Source: CAD feature listing. Evaluate the final solid. Frame: model axes, mm. Face numbers are marked on the shaded views. Coordinates: 2 decimals unless noted, no trailing zeros. Loops run counter-clockwise (first coordinate to the right, second up) from the corner with the lowest first, then second, coordinate; pieces in that order, holes last. Notation, with made-up numbers: (84.5, -21) -> (141.5, -21) arc R12 cw to (141.5, -4) -> close; hole circle Ø2 at (-13.75, -24.5). An arc over 180 degrees is marked (long way). Answer as a JSON object with one key per item and string values. Group by question number.
from build123d import *

# Parameters (mm, degrees)
SKETCH1_R           = 1.6
BOSS_EXTRUDE1_DEPTH = 3.175


with BuildPart() as part:
    # Sketch1 → Boss-Extrude1 (new body)
    with BuildSketch(Plane.XY):
        Polygon((0, 0), (43.867513459, 0), (43.867513459, -50), (28.867513459, -50), align=None)
        with Locations((36.367513459, -5)):
            Circle(SKETCH1_R, mode=Mode.SUBTRACT)
        with Locations((36.367513459, -45)):
            Circle(SKETCH1_R, mode=Mode.SUBTRACT)
        with Locations((11.547005384, -5)):
            Circle(SKETCH1_R, mode=Mode.SUBTRACT)
        with Locations((25.867513459, -29.803847577)):
            Circle(SKETCH1_R, mode=Mode.SUBTRACT)
    extrude(amount=BOSS_EXTRUDE1_DEPTH)


solid = part.part
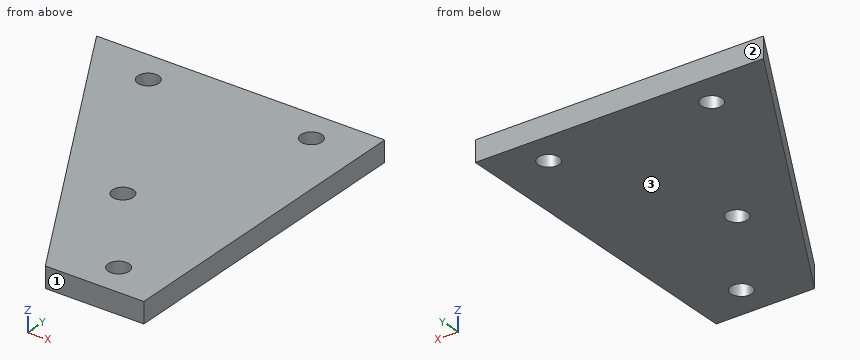
1. Section query C-C on x = 26. Return loops of the section in (y, z) (3 decimals), then the cut area to 3 significant figures.
2. Pin query (flat end, axial travel): pin 1 Ø1.9 at (x, y) = (11.55, -5) entering from -Z. Return the tip coordinate at first contact, or that it passes through.
3. Section query D-D on y = -45. Return loops of the section in (x, z) (3 decimals), then the cut area to 3 significant figures.
4. Section query B-B on y = -4. Return loops of the section in (x, z) (3 decimals), then the cut area to 3 significant figures.
5. Ray query, L1, parallel to Y at x = 36, z = 2.8; L2, parallel to Y at x = 37.5, z = 1.65; L3, parallel to X at y = -46, z = 2.85. Return the intervals inside material, ascending.
6. Mould query, pull axis Y, two halves, no side actions, for the marked faces 1, 2 and 3. Classes: pulls with the +Y half, pulls with the -Y half, needs draft (parallel to the pull), parting line crosses it, or undercut.
7. Section query A-A on z = 2.1. Return loops of the section in (x, y), then the cut area to 3 significant figures.
Solved:
{
 "1": {"outline": "(-45.033, 0) -> (-31.398, 0) -> (-31.398, 3.175) -> (-45.033, 3.175) -> close; (-28.209, 0) -> (0, 0) -> (0, 3.175) -> (-28.209, 3.175) -> close", "area": "133 mm^2"},
 "2": {"pin 1": "through"},
 "3": {"outline": "(25.981, 0) -> (34.768, 0) -> (34.768, 3.175) -> (25.981, 3.175) -> close; (37.968, 0) -> (43.868, 0) -> (43.868, 3.175) -> (37.968, 3.175) -> close", "area": "46.6 mm^2"},
 "4": {"outline": "(2.309, 0) -> (10.298, 0) -> (10.298, 3.175) -> (2.309, 3.175) -> close; (12.796, 0) -> (35.119, 0) -> (35.119, 3.175) -> (12.796, 3.175) -> close; (37.617, 0) -> (43.868, 0) -> (43.868, 3.175) -> (37.617, 3.175) -> close", "area": "116 mm^2"},
 "5": {"L1": "-50 to -46.56, -43.44 to -6.56, -3.44 to 0", "L2": "-50 to -46.13, -43.87 to -6.13, -3.87 to 0", "L3": "26.56 to 35.12, 37.62 to 43.87"},
 "6": {"face 1": "pulls with the -Y half", "face 2": "pulls with the +Y half", "face 3": "needs draft"},
 "7": {"outline": "(0, 0) -> (28.87, -50) -> (43.87, -50) -> (43.87, 0) -> close; hole circle Ø3.2 at (11.55, -5); hole circle Ø3.2 at (25.87, -29.8); hole circle Ø3.2 at (36.37, -45); hole circle Ø3.2 at (36.37, -5)", "area": "1,440 mm^2"}
}
